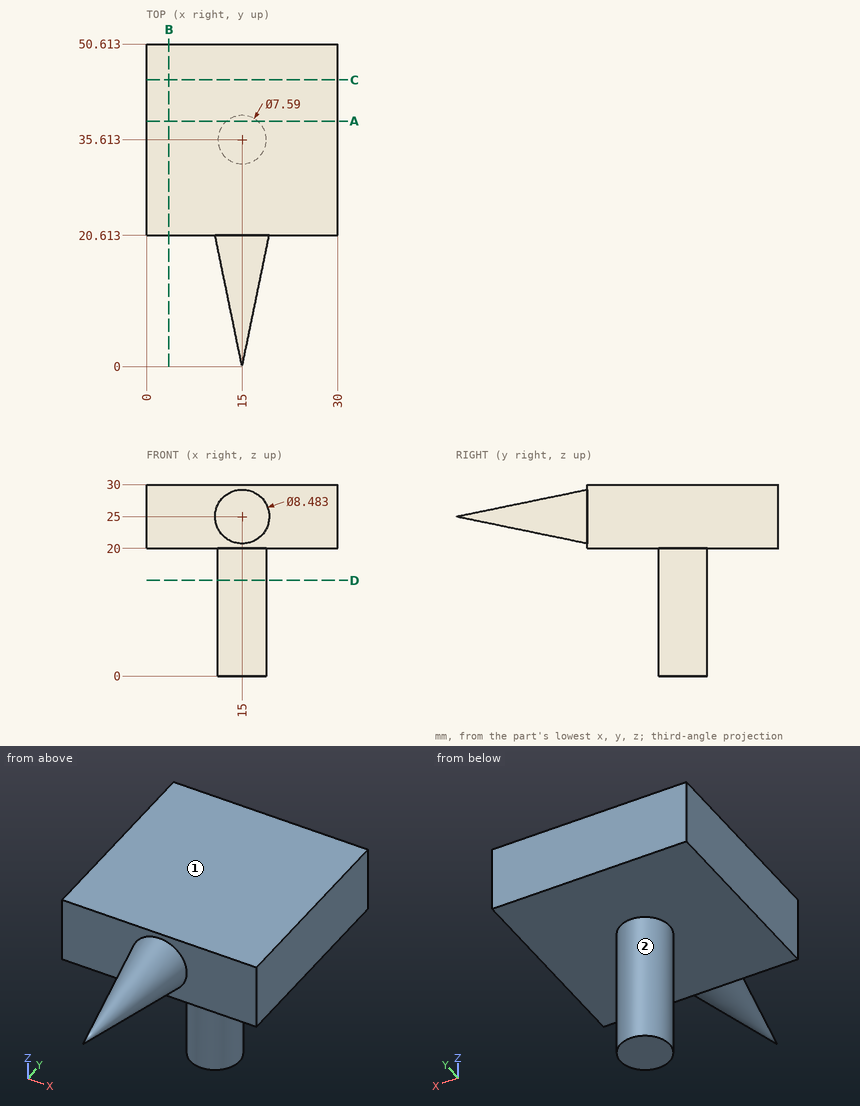
Input: dimensioned drawing with shaded views. Units: mm. Origin: part minimum x, y, z. A direction names the side the tool comes from. Round coordinates to 2 decimals unless told otherwise and drop trailing zeros. Order: outer loops, then holes, each group sorted by start corner. A loop starts at its lowest first (then second) coordinate and runs counter-clockwise, first axis right, second up.
1. Material intervals for line 1 (Z direction, x = 19, y = 47); line 2 (Y direction, x = 20.25, z = 24.5); line 3 (Y direction, x = 16, z = 6.75) (1 decimal), sorted ascending.
The answers:
line 1: z = 20 to 30
line 2: y = 20.61 to 50.61
line 3: y = 32 to 39.3
2. Cut plane D-D, the plane z = 15. Output: boundary loops of the cut face in (x, y) (1 decimal).
The answers:
outline: circle Ø7.6 at (15, 35.6)
3. Cut plane C-C, the plane y = 45. Output: boundary loops of the cut face in (x, z), then the cut area to 3 significant figures.
The answers:
outline: (0, 20) - (30, 20) - (30, 30) - (0, 30) - close
area: 300 mm2
4. Pin query (flat end, axial travel): P1, Ø2, axis at x = 21, z = 13.5, coming from the -Y side; P2, Ø8, axis at x = 4, y = 35.5, coming from the -Z side; P3, Ø1, axis at y = 11, z = 25, coming from the -X side. Return the tip coordinate at first contact, or that it passes through.
The answers:
P1: passes through
P2: stops at z = 20
P3: stops at x = 12.63
5. Cut plane A-A, the plane y = 38.5. Output: boundary loops of the cut face in (x, z).
The answers:
outline: (0, 20) - (12.54, 20) - (12.54, 0) - (17.46, 0) - (17.46, 20) - (30, 20) - (30, 30) - (0, 30) - close
6. Cut plane B-B, the plane x = 3.5. Output: boundary loops of the cut face in (y, z).
The answers:
outline: (20.61, 20) - (50.61, 20) - (50.61, 30) - (20.61, 30) - close
7. Set-up query: the marked faces 1 and 2. Return all of +Z, -Z, +X, -X, +Y, -Y with unobstructed straight access to the full face (end or side cutting, diameter ignored); none if empty.
The answers:
face 1: +Z, +X, -X, +Y, -Y
face 2: -Z
